Verification items for the finished model (mm, model axes). A direction names the side the tool comes from. Give positions to 0.01 mm unless a question says otherwise; leave off trailing zeros. Write each loop counter-clockwise with the first axis right and the second up, starting at its lowest first coordinate (ties: lowest second). Pieces come first, ordered by that corner, then holes. Notation, with made-up numbers: M 85.5,24.5 L 118.5,24.5 A21 cw 118.5,34.5 Z; hole C -20,67.25 d1. An arc over 180 degrees is marked long. Answer as a JSON object with one key per item and string values.
```python
from build123d import *

# Parameters (mm, degrees)
SKETCH1_R           = 7.9375
BOSS_EXTRUDE1_DEPTH = 6.35


with BuildPart() as part:
    # Sketch1 → Boss-Extrude1 (new body)
    with BuildSketch(Plane.XY):
        with BuildLine():
            Line((-40.005, -31.35), (40.005, -31.35))
            Line((40.005, -31.35), (40.005, -21.35))
            Line((40.005, -21.35), (20.6375, -21.35))
            Line((20.6375, -21.35), (20.6375, 0))
            ThreePointArc((20.6375, 0), (0, 20.6375), (-20.6375, 0))
            Line((-20.6375, 0), (-20.6375, -21.35))
            Line((-20.6375, -21.35), (-40.005, -21.35))
            Line((-40.005, -21.35), (-40.005, -31.35))
        make_face()
        Circle(SKETCH1_R, mode=Mode.SUBTRACT)
    extrude(amount=BOSS_EXTRUDE1_DEPTH)


solid = part.part
```
1) Section check D-D on x = -26. Record the boundary of the cut face in (y, z), and give its area (3 significant figures).
Completed:
{"outline": "M -31.35,0 L -21.35,0 L -21.35,6.35 L -31.35,6.35 Z", "area": "63.5 mm2"}
2) Section check C-C on y = -20. Record the boundary of the cut face in (x, z).
Completed:
{"outline": "M -20.64,0 L 20.64,0 L 20.64,6.35 L -20.64,6.35 Z"}
3) Go/stop test with a flat-tipped pin: pin 1 (3 mm diameter, centred on y = -13.5, z = 1, fed in from +X). Record where the tip stops, or that it passes through.
Completed:
{"pin 1": "stops at x = 20.64"}
4) Section check A-A on x = 0. Record the boundary of the cut face in (y, z).
Completed:
{"outline": "M -31.35,0 L -7.94,0 L -7.94,6.35 L -31.35,6.35 Z; M 7.94,0 L 20.64,0 L 20.64,6.35 L 7.94,6.35 Z"}
5) Release check for a two-part mould opening along Y. For faces 1 (the face through (-30, -21.35, 3)), 2 (the face through (-1.72, -7.75, 3.13)), 3 (the face through (-1, -31.35, 3)), 4 (the face through (-1, -11, 6.35)) record: pulls with the +Y half, pulls with the -Y half, needs draft (parallel to the pull), parting line crosses it, or undercut.
Completed:
{"face 1": "pulls with the +Y half", "face 2": "undercut", "face 3": "pulls with the -Y half", "face 4": "needs draft"}
6) Thickness scan on L1, parallel to Y at x = 0, z = 4.5; L2, parallel to Y at x = -21.5, z = 2; L3, parallel to X at y = -2, z = 4. Record the ranges inside material, lowest first.
Completed:
{"L1": "y = -31.35 to -7.94, 7.94 to 20.64", "L2": "y = -31.35 to -21.35", "L3": "x = -20.64 to -7.68, 7.68 to 20.64"}
7) Access from +Z, -Z, +X, -X, +Y, -Y to the whole of each face (thin tool, end or side, straight path). Record for faces 5 (the face through (-40.005, -26, 3)), 6 (the face through (20.638, -11, 3)), 7 (the face through (-20.638, -11, 3)).
Completed:
{"face 5": "+Z, -Z, -X, +Y, -Y", "face 6": "+Z, -Z, +X, +Y", "face 7": "+Z, -Z, -X, +Y"}
